Design review of the part built by this model. Coordinates are the model's own, in mm. Face numbers are marked on the shaded views. Give positions to 0.01 mm unless a question says otherwise; leave off trailing zeros. Loops run counter-clockwise (first coordinate to the right, second up) from the corner with the lowest first, then second, coordinate; pieces in that order, holes last. Notation, with made-up numbers: (-32, 7) -> (-13, 7) arc R17 ccw to (-13, 18) -> close; hole circle Ø3 at (47.25, 56.5). An arc over 180 degrees is marked (long way). Answer in a Markdown table with one row per item. Add a question column.
(1) Consider section A-A on y = 50.29. Write out the cut boundary in (x, z).
(2) Consider section B-B on x = 14.25. Count the separate pieces of the cut face and the enclosed holes in it, then the cut area to 3 significant figures.
(3) Draft analysis for pull direction X (two halves, no side actions). For the marked faces 1, 2, 3 and 4, state which applies: +X half, -X half, draft (parallel to the pull), parting line (faces both ways), or undercut.
(4) Consider section D-D on z = -9.5. Write out the cut boundary in (x, y), then the cut area to 3 significant figures.
(5) For pin 1 (5 mm diameter, centred on x = 20, y = 35, fed in from -Z); pin 2 (1.3 mm diameter, centred on x = 5.5, y = 49.5, fed in from +Z), all flat-tipped, find the tip position at first contact; note any pin that passes through.
(6) Consider section C-C on z = -21.5. Write out the cut boundary in (x, y), then the cut area to 3 significant figures.
(7) For line 1 (Y direction, x = 4.5, z = -2.75); line 2 (X direction, y = 4.57, z = -3.5); line 3 (X direction, y = 14, z = -1.25), list the stretches that pass through material, from the lowest coordinate up.
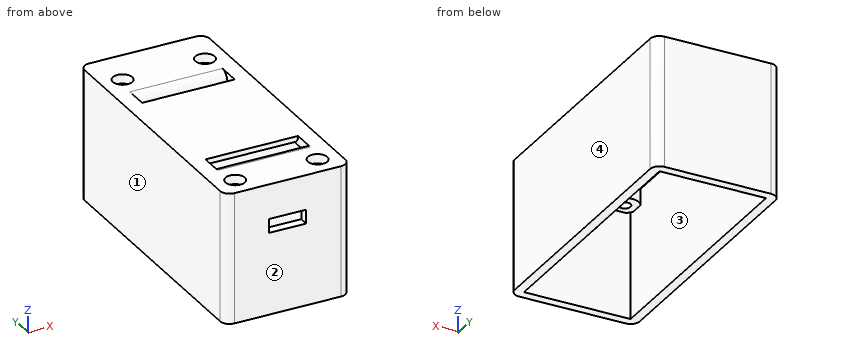
Autodesk Inventor part; units mm, degrees
ref_plane "YZ Plane" through (0, 0, 0) normal (1, 0, 0) x (0, 1, 0)
ref_plane "XZ Plane" through (0, 0, 0) normal (0, 1, 0) x (-1, 0, 0)
ref_plane "XY Plane" through (0, 0, 0) normal (0, 0, 1) x (1, 0, 0)
sketch "Skizze1" plane through (0, 0, 0) normal (0, 0, 1) x (1, 0, 0)
  line L0 (0, 0) -> (27, 0)
  line L1 (27, 0) -> (27, 59)
  line L2 (27, 59) -> (0, 59)
  line L3 (0, 59) -> (0, 0)
  dimension "d0" = 27
  dimension "d1" = 59
extrude "Extrusion1" add sketch "Skizze1" against normal blind 28.2
sketch "Skizze2" plane through (0, 0, -28.2) normal (0, 0, -1) x (-1, 0, 0)
  line L0 (-2, 57) -> (-25, 57)
  line L1 (-25, 57) -> (-25, 2)
  line L2 (-25, 2) -> (-2, 2)
  line L3 (-2, 2) -> (-2, 57)
  line L4 (0, 59) -> (-27, 59) construction
  line L5 (-27, 59) -> (-27, 0) construction
  point P0 (0, 0)
  dimension "d4" = 2
  dimension "d5" = 2
  dimension "d6" = 2
  dimension "d7" = 2
extrude "Extrusion2" cut sketch "Skizze2" against normal blind 26.2
sketch "Skizze3" plane through (0, 0, -2) normal (0, 0, -1) x (-1, 0, 0)
  circle A0 centre (-4.61, 4.57) radius 3
  line L0 (-2, 2) -> (-25, 2) construction
  line L1 (-2, 57) -> (-2, 2) construction
  circle A1 centre (-22.39, 4.57) radius 3
  circle A2 centre (-4.61, 50.29) radius 3
  circle A3 centre (-22.39, 50.29) radius 3
  line L2 (-4.61, 4.57) -> (-22.39, 4.57) construction
  point P0 (0, 0)
  point P1 (-13.5, 4.57)
  point P2 (-13.5, 2)
  dimension "d13" = 6
  dimension "d18" = 17.78
  dimension "d21" = 45.72
  dimension "d66" = 2.57
extrude "Extrusion4" add sketch "Skizze3" along normal blind 3.5
sketch "Skizze7" plane through (4.61, 50.29, -5.5) normal (0, 0, -1) x (0, -1, 0)
  circle A0 centre (0, 0) radius 3 construction
  circle A1 centre (0, -17.78) radius 3 construction
  circle A2 centre (45.72, -17.78) radius 3 construction
  circle A3 centre (45.72, 0) radius 3 construction
  point P0 (50.29, 4.61)
  point P1 (0, -17.78)
  point P2 (45.72, 0)
hole "Bohrung2" at (4.61, 50.29, -5.5) at (22.39, 50.29, -5.5) at (22.39, 4.57, -5.5) at (4.61, 4.57, -5.5) direction (0, 0, 1) diameter 2.5 end through all
sketch "Skizze8" plane through (0, 0, -2) normal (0, 0, -1) x (-1, 0, 0)
  line L0 (-3.5, 11.57) -> (-23.5, 11.57)
  line L1 (-23.5, 11.57) -> (-23.5, 14.57)
  line L2 (-23.5, 14.57) -> (-3.5, 14.57)
  line L3 (-3.5, 14.57) -> (-3.5, 11.57)
  line L4 (-2, 2) -> (-25, 2) construction
  circle A0 centre (-4.61, 4.57) radius 3 construction
  line L5 (-3.5, 43.29) -> (-23.5, 43.29)
  line L6 (-23.5, 43.29) -> (-23.5, 40.29)
  line L7 (-23.5, 40.29) -> (-3.5, 40.29)
  line L8 (-3.5, 40.29) -> (-3.5, 43.29)
  circle A1 centre (-4.61, 50.29) radius 3 construction
  point P0 (0, 0)
  point P1 (-13.5, 11.57)
  point P2 (-13.5, 2)
  point P3 (-13.5, 2)
  point P4 (-13.5, 40.29)
  dimension "d43" = 3
  dimension "d44" = 20
  dimension "d45" = 4
  dimension "d46" = 3
  dimension "d47" = 20
  dimension "d48" = 4
extrude "Extrusion5" cut sketch "Skizze8" against normal through all
sketch "Skizze9" plane through (0, 0, 0) normal (0, -1, 0) x (1, 0, 0)
  line L0 (2, -5.5) -> (3.0624, -5.5) construction
  line L1 (17.5, -10.5) -> (9.5, -10.5)
  line L2 (9.5, -10.5) -> (9.5, -7.5)
  line L3 (9.5, -7.5) -> (17.5, -7.5)
  line L4 (17.5, -7.5) -> (17.5, -10.5)
  line L5 (0, 0) -> (27, 0) construction
  point P0 (13.5, -7.5)
  point P1 (13.5, 0)
  dimension "d54" = 8
  dimension "d55" = 3
  dimension "d56" = 2
extrude "Extrusion6" cut sketch "Skizze9" against normal up to surface (2 mm away)
sketch "Skizze10" plane through (0, 0, 0) normal (0, 0, 1) x (1, 0, 0)
  circle A0 centre (4.61, 4.57) radius 1.25 construction
  circle A1 centre (22.39, 4.57) radius 1.25 construction
  circle A2 centre (22.39, 50.29) radius 1.25 construction
  circle A3 centre (4.61, 50.29) radius 1.25 construction
  point P0 (0, 0)
hole "Bohrung3" at (4.61, 4.57, 0) at (22.39, 4.57, 0) at (22.39, 50.29, 0) at (4.61, 50.29, 0) direction (0, 0, -1) diameter 2.5 end through all counterbore diameter 4.2 counterbore depth 2
fillet "Rundung1" radius 2 4 edges at (27, 0, -14.1) (0, 0, -14.1) (0, 59, -14.1) (27, 59, -14.1)
fillet "Rundung2" radius 2 2 edges at (13.5, 14.57, -2) (13.5, 40.29, -2)
fillet "Rundung3" radius 2 2 edges at (13.5, 11.57, 0) (13.5, 43.29, 0)
properties part number "bottom"
Values follow:
| question | item | result |
|---|---|---|
| 1 | outline | (0, -28.2) -> (2, -28.2) -> (2, -5.5) -> (3.36, -5.5) -> (3.36, -2) -> (2.51, -2) -> (2.51, 0) -> (0, 0) -> close; (5.86, -5.5) -> (7.61, -5.5) -> (7.61, -2) -> (19.39, -2) -> (19.39, -5.5) -> (21.14, -5.5) -> (21.14, -2) -> (20.29, -2) -> (20.29, 0) -> (6.71, 0) -> (6.71, -2) -> (5.86, -2) -> close; (23.64, -5.5) -> (25, -5.5) -> (25, -28.2) -> (27, -28.2) -> (27, 0) -> (24.49, 0) -> (24.49, -2) -> (23.64, -2) -> close |
| 2 | separate pieces | 4 |
| 2 | enclosed holes | 0 |
| 2 | area | 201 mm2 |
| 3 | face 1 | -X half |
| 3 | face 2 | draft |
| 3 | face 3 | undercut |
| 3 | face 4 | +X half |
| 4 | outline | (0, 2) arc R2 ccw to (2, 0) -> (9.5, 0) -> (9.5, 2) -> (2, 2) -> (2, 57) -> (25, 57) -> (25, 2) -> (17.5, 2) -> (17.5, 0) -> (25, 0) arc R2 ccw to (27, 2) -> (27, 57) arc R2 ccw to (25, 59) -> (2, 59) arc R2 ccw to (0, 57) -> close |
| 4 | area | 309 mm2 |
| 5 | pin 1 | z = -2 |
| 5 | pin 2 | z = -2 |
| 6 | outline | (0, 2) arc R2 ccw to (2, 0) -> (25, 0) arc R2 ccw to (27, 2) -> (27, 57) arc R2 ccw to (25, 59) -> (2, 59) arc R2 ccw to (0, 57) -> close; hole (2, 2) -> (25, 2) -> (25, 57) -> (2, 57) -> close |
| 6 | area | 325 mm2 |
| 7 | line 1 | 0 to 3.32, 5.82 to 7.57, 47.29 to 49.04, 51.54 to 53.29, 57 to 59 |
| 7 | line 2 | 0 to 3.36, 5.86 to 7.61, 19.39 to 21.14, 23.64 to 27 |
| 7 | line 3 | 0 to 3.5, 23.5 to 27 |
